from build123d import *

# Parameters (mm, degrees)
F0_R           = 15.875
F0_R_2         = 9.525
F1_DEPTH       = 12.7
F5_DEPTH       = 25.4
F7_DEPTH       = 25.4
F9_DEPTH       = 6.35
F11_W          = 31.75
F11_H          = 19.05
F12_DEPTH      = 9.525
F14_END_RADIUS = 15.875
F13_W          = 3.175
F13_H          = 19.05
F14_REACH      = 79.7657711337
F16_DEPTH      = 25.4
F17_R          = 9.525
F18_DEPTH      = 11.176
F19_W          = 22.225
F19_H          = 7.9375
F20_DEPTH      = 8.001
F21_R          = 1.7272
F22_DEPTH      = 101.6


with BuildPart() as f1:
    # F0 (on Top) → F1 (new body)
    with BuildSketch(Plane.XY):
        Circle(F0_R)
        Circle(F0_R_2, mode=Mode.SUBTRACT)
    extrude(amount=F1_DEPTH)

    # F4 (on face) → F5 (cut)
    with BuildSketch(Plane(origin=(0, 0, 0), x_dir=(-0.7071067812, 0.7071067812, 0), z_dir=(0.7071067812, 0.7071067812, 0))):
        with BuildLine():
            ThreePointArc((0, 6.1468), (1.2213148325, 6.6526851675), (1.7272, 7.874))
            ThreePointArc((1.7272, 7.874), (1.2213148325, 9.0953148325), (0, 9.6012))
            Line((0, 9.6012), (0, 6.1468))
        make_face()
        with BuildLine():
            Line((0, 6.1468), (0, 9.6012))
            ThreePointArc((0, 9.6012), (-1.7272, 7.874), (0, 6.1468))
        make_face()
    extrude(amount=-F5_DEPTH, mode=Mode.SUBTRACT)

    # F6 (on face) → F7 (cut)
    with BuildSketch(Plane(origin=(0, 0, 0), x_dir=(-0.7071067812, -0.7071067812, 0), z_dir=(-0.7071067812, 0.7071067812, 0))):
        with BuildLine():
            ThreePointArc((0, 6.1468), (1.2213148325, 6.6526851675), (1.7272, 7.874))
            ThreePointArc((1.7272, 7.874), (1.2213148325, 9.0953148325), (0, 9.6012))
            Line((0, 9.6012), (0, 6.1468))
        make_face()
        with BuildLine():
            Line((0, 6.1468), (0, 9.6012))
            ThreePointArc((0, 9.6012), (-1.7272, 7.874), (0, 6.1468))
        make_face()
    extrude(amount=F7_DEPTH, mode=Mode.SUBTRACT)

    # F8 (on face) → F9 (join)
    with BuildSketch(Plane(origin=(0, 0, 0), x_dir=(1, 0, 0), z_dir=(0, 0, -1))):
        with BuildLine():
            Line((54.102, 15.875), (0, 15.875))
            ThreePointArc((0, 15.875), (11.2253201513, 11.2253201513), (15.875, 0))
            ThreePointArc((15.875, 0), (11.2253201513, -11.2253201513), (0, -15.875))
            Line((0, -15.875), (54.102, -15.875))
            Line((54.102, -15.875), (54.102, 15.875))
        make_face()
    extrude(amount=-F9_DEPTH)

    # F11 (on offset) → F12 (join)
    with BuildSketch(Plane.YZ.offset(54.102)):
        with Locations((0, 15.875)):
            Rectangle(F11_W, F11_H)
        with BuildLine():
            ThreePointArc((15.875, 25.4), (0, 41.275), (-15.875, 25.4))
            Line((-15.875, 25.4), (15.875, 25.4))
        make_face()
    extrude(amount=-F12_DEPTH)

    f14_end = (Plane(origin=(0, 0, 6.35), x_dir=(-1, 0, 0), z_dir=(0, 0, -1)) * Cylinder(F14_END_RADIUS, 333.9846154871, mode=Mode.PRIVATE)).faces().sort_by_distance((-15.875, 0, 6.35))[0]
    # F13 (on face) → F14 (join, up to the whole of a round face its end follows)
    with BuildSketch(Plane(origin=(44.577, 0, 0), x_dir=(0, -1, 0), z_dir=(-1, 0, 0))):
        with Locations((-1.5875, 15.875)):
            Rectangle(F13_W, F13_H)
        with Locations((1.5875, 15.875)):
            Rectangle(F13_W, F13_H)
    f14_long = extrude(amount=F14_REACH, mode=Mode.PRIVATE)
    add(split(f14_long, bisect_by=f14_end, keep=Keep.ALL, mode=Mode.PRIVATE).solids().sort_by_distance((44.577, 0, 15.875))[0])

    # F15 (on face) → F16 (cut)
    with BuildSketch(Plane.XZ.offset(3.175)):
        with BuildLine():
            Line((19.3865235489, 10.5133005292), (44.577, 25.4))
            Line((44.577, 25.4), (15.5542598667, 25.4))
            Line((15.5542598667, 25.4), (15.5542598667, 12.7))
            ThreePointArc((15.5542598667, 12.7), (16.8354409267, 10.4938778646), (19.3865235489, 10.5133005292))
        make_face()
    extrude(amount=-F16_DEPTH, mode=Mode.SUBTRACT)

    # F17 (on face) → F18 (join)
    with BuildSketch(Plane.YZ.offset(54.102)):
        with Locations((0, 25.4)):
            Circle(F17_R)
    extrude(amount=F18_DEPTH)

    # F19 (on face) → F20 (cut)
    with BuildSketch(Plane.YZ.offset(54.102)):
        with Locations((0, 10.31875)):
            Rectangle(F19_W, F19_H)
    extrude(amount=-F20_DEPTH, mode=Mode.SUBTRACT)

    # F21 (on face) → F22 (cut)
    with BuildSketch(Plane.XZ.offset(15.875)):
        with Locations((50.927, 10.287)):
            Circle(F21_R)
    extrude(amount=-F22_DEPTH, mode=Mode.SUBTRACT)


solid = f1.part
Model file for the job. Use its own axes, mm. A direction names the side the tool comes from. Give positions to 0.01 mm unless a question says otherwise; leave off trailing zeros. Loops run counter-clockwise (first coordinate to the right, second up) from the corner with the lowest first, then second, coordinate; pieces in that order, holes last. Notation, with made-up numbers: (20.5, 13.5) - (77.5, 13.5) arc R23 cw to (77.5, 43.5) - close; hole circle Ø10 at (-22.5, 9). An arc over 180 degrees is marked (long way). Use one line per item in the form item = value.
(1) Pull direction Y, two halves, no side cores. Call faces 1 (the face through (8.8, -3.65, 6.26)), 2 (the face through (27, 9, 6.35)), 3 (the face through (-15.86, 0.65, 7.67)): pulls with the +Y half, pulls with the -Y half, needs draft (parallel to the pull), parting line crosses it, or undercut.
Determined:
face_1 = undercut
face_2 = needs draft
face_3 = parting line crosses it
(2) 3-axis set-ups, long thin cutter, end or side, ignore diameter. For faces 4 (the face through (27, -10, 6.35)), 5 (the face through (33, -15.875, 4)), 6 (the face through (50, 0, 6.35)), 7 (the face through (44.577, -4, 24)), 8 (the face through (33, 3.175, 14)): which of +Z, -Z, +X, -X, +Y, -Y reach the whole face in a straight line?
Determined:
face_4 = +Z, -Y
face_5 = +Z, -Z, +X, -X, -Y
face_6 = +X
face_7 = +Z
face_8 = +Z, +Y
(3) Drill centre lines: L1, parallel to Y at x = 48.5, z = 8 (1 decimal); L2, parallel to Y at x = 0, z = 6.75 (3 decimals); L3, parallel to X at y = -1.5, z = 12.5. Where is each one in solid material? Low to high.
Determined:
L1 = -15.9 to -11.1, 11.1 to 15.9
L2 = -15.875 to -9.525, 9.525 to 15.875
L3 = -15.8 to -9.41, 9.41 to 15.56, 22.75 to 46.1
(4) Drop flat-ended pins along their axis: P1, Ø11.5, axis at x = 0, y = 0, coming from the -Z side (3 decimals); P2, Ø6.5, axis at x = 12.5, y = 9.5, coming from the +Z side; P3, Ø3, axis at x = 35.5, z = 20, coming from the +Y side (3 decimals); P4, Ø1.5, axis at x = 49.5, z = 33.5, coming from the +Y side. Give the stop position or say it passes through.
Determined:
P1 = through
P2 = 12.7
P3 = 3.175
P4 = 14.07
(5) Cut at C-C (z = 24.5). Give the cut face in (x, y) (3 decimals), then the cut area to 3 significant figures.
Determined:
outline = (43.054, -3.175) - (44.577, -3.175) - (44.577, -15.875) - (54.102, -15.875) - (54.102, -9.482) - (65.278, -9.482) - (65.278, 9.482) - (54.102, 9.482) - (54.102, 15.875) - (44.577, 15.875) - (44.577, 3.175) - (43.054, 3.175) - close
area = 524 mm^2
(6) Cut at B-B (x = 3.5). Give the cut face in (y, z) (3 decimals), then the cut area to 3 significant figures.
Determined:
outline = (-15.875, 0) - (-8.859, 0) - (-8.859, 12.7) - (-15.484, 12.7) - (-15.484, 6.35) - (-15.875, 6.35) - close; (8.859, 0) - (15.875, 0) - (15.875, 6.35) - (15.484, 6.35) - (15.484, 12.7) - (8.859, 12.7) - close
area = 173 mm^2
(7) Cut at D-D (y = 13.5). Give the cut face in (x, z), then the cut area to 3 significant figures.
Determined:
outline = (-8.35, 0) - (54.1, 0) - (54.1, 33.75) - (44.58, 33.75) - (44.58, 6.35) - (8.35, 6.35) - (8.35, 12.7) - (-8.35, 12.7) - close; hole circle Ø3.45 at (50.93, 10.29)
area = 754 mm^2
